```python
from build123d import *

# Parameters (mm, degrees)
SKETCH1_W                  = 120
SKETCH1_H                  = 50
BOSS_EXTRUDE1_DEPTH        = 160
SHELL1_T                   = -5
CUT_EXTRUDE2_REACH         = 174.699
SKETCH4_W                  = 72
SKETCH4_H                  = 39
SKETCH5_W                  = 80
SKETCH5_H                  = 43.5
CUT_EXTRUDE3_DEPTH         = 1
CUT_EXTRUDE4_REACH         = 174.699
SKETCH7_R                  = 10.054878977
CUT_EXTRUDE5_DEPTH         = 1
CUT_EXTRUDE6_REACH         = 203.556
SKETCH9_R                  = 1.35
CHAMFER1_SIZE              = 1.5
SKETCH10_W                 = 12
SKETCH10_H                 = 28
CUT_EXTRUDE7_DEPTH         = 2
LPATTERN1_COUNT            = 2
LPATTERN1_PITCH            = 50
CHAMFER1_OF_LPATTERN1_SIZE = 1.5
SKETCH11_W                 = 19.287715199
SKETCH11_H                 = 31.517777442
CUT_EXTRUDE8_DEPTH         = 202.556443707
SKETCH12_W                 = 24.096142941
SKETCH12_H                 = 37.033540034
CUT_EXTRUDE9_DEPTH         = 3
CUT_EXTRUDE10_REACH        = 174.699
SKETCH13_W                 = 24.602100194
SKETCH13_H                 = 34.536068778
SKETCH2_W                  = 80
SKETCH2_H                  = 57.520884572
CUT_EXTRUDE1_DEPTH         = 177.705970471


with BuildPart() as part:
    # Sketch1 → Boss-Extrude1 (new body)
    with BuildSketch(Plane.XY):
        Rectangle(SKETCH1_W, SKETCH1_H)
    extrude(amount=-BOSS_EXTRUDE1_DEPTH)

    # Shell1
    shell1_openings = [part.faces().sort_by_distance(p)[0] for p in [
        (-60, 0, -80),
        (0, 25, -80),
    ]]
    offset(amount=SHELL1_T, openings=shell1_openings, kind=Kind.INTERSECTION)

    # Sketch4 → Cut-Extrude2 (cut, up to next)
    with BuildSketch(Plane.XY, mode=Mode.PRIVATE) as cut_extrude2_sk1:
        with Locations((-7.752822836, -0.864806595)):
            Rectangle(SKETCH4_W, SKETCH4_H)
    cut_extrude2_tool1 = extrude(cut_extrude2_sk1.sketch, amount=-CUT_EXTRUDE2_REACH, mode=Mode.PRIVATE) & part.part
    add(cut_extrude2_tool1.solids().sort_by_distance((-7.752823, -0.864807, 0))[0], mode=Mode.SUBTRACT)

    # Sketch5 → Cut-Extrude3 (cut)
    with BuildSketch(Plane.XY):
        with Locations((-7.752822836, -0.864806595)):
            Rectangle(SKETCH5_W, SKETCH5_H)
    extrude(amount=-CUT_EXTRUDE3_DEPTH, mode=Mode.SUBTRACT)

    # Sketch6 → Cut-Extrude4 (cut, up to next)
    with BuildSketch(Plane.XY, mode=Mode.PRIVATE) as cut_extrude4_sk1:
        with BuildLine():
            Line((51.25624878, 9.193705725), (51.25624878, 16.439437846))
            ThreePointArc((51.25624878, 16.439437846), (44.123588582, 20.816571785), (36.990928383, 16.439437846))
            Line((36.990928383, 16.439437846), (36.990928383, 9.193705725))
            ThreePointArc((36.990928383, 9.193705725), (44.123588582, 4.816571785), (51.25624878, 9.193705725))
        make_face()
    cut_extrude4_tool1 = extrude(cut_extrude4_sk1.sketch, amount=-CUT_EXTRUDE4_REACH, mode=Mode.PRIVATE) & part.part
    cut_extrude4 = cut_extrude4_tool1.solids().sort_by_distance((44.123589, 12.816572, 0))[0]
    add(cut_extrude4, mode=Mode.SUBTRACT)

    # Sketch7 → Cut-Extrude5 (cut)
    with BuildSketch(Plane.XY):
        with Locations((44.123588582, 12.816571785)):
            Circle(SKETCH7_R)
    cut_extrude5 = extrude(amount=-CUT_EXTRUDE5_DEPTH, mode=Mode.SUBTRACT)

    # Mirror1: Cut-Extrude4, Cut-Extrude5 mirrored; each copy of Cut-Extrude4 runs up to whatever stops it at its own place
    mirror1_before = part.part  # the part as the pattern finds it: every copy runs up to it
    mirror1_cut_extrude4_long = extrude(cut_extrude4_sk1.sketch, amount=-CUT_EXTRUDE4_REACH, mode=Mode.PRIVATE)
    mirror1_cut_extrude4_tool = mirror1_cut_extrude4_long.mirror(Plane.ZX) & mirror1_before
    add(mirror1_cut_extrude4_tool.solids().sort_by_distance((44.123589, -12.816572, 0))[0], mode=Mode.SUBTRACT)
    add(cut_extrude5.mirror(Plane.ZX), mode=Mode.SUBTRACT)

    # Sketch9 → Cut-Extrude6 (cut, up to next)
    with BuildSketch(Plane(origin=(60, 0, 0), x_dir=(0, 0, -1), z_dir=(1, 0, 0)), mode=Mode.PRIVATE) as cut_extrude6_sk1:
        with Locations((34.250404533, 14.202757041)):
            Circle(SKETCH9_R)
    cut_extrude6_tool1 = extrude(cut_extrude6_sk1.sketch, amount=-CUT_EXTRUDE6_REACH, mode=Mode.PRIVATE) & part.part
    # Sketch9 → Cut-Extrude6 (cut, up to next)
    with BuildSketch(Plane(origin=(60, 0, 0), x_dir=(0, 0, -1), z_dir=(1, 0, 0)), mode=Mode.PRIVATE) as cut_extrude6_sk2:
        with Locations((34.250404533, -8.297242959)):
            Circle(SKETCH9_R)
    cut_extrude6_tool2 = extrude(cut_extrude6_sk2.sketch, amount=-CUT_EXTRUDE6_REACH, mode=Mode.PRIVATE) & part.part
    # Sketch9 → Cut-Extrude6 (cut, up to next)
    with BuildSketch(Plane(origin=(60, 0, 0), x_dir=(0, 0, -1), z_dir=(1, 0, 0)), mode=Mode.PRIVATE) as cut_extrude6_sk3:
        with BuildLine():
            Line((29.950404533, -5.047242959), (38.550404533, -5.047242959))
            Line((38.550404533, -5.047242959), (38.550404533, 7.952757041))
            ThreePointArc((38.550404533, 7.952757041), (37.671724876, 10.074077384), (35.550404533, 10.952757041))
            Line((35.550404533, 10.952757041), (32.950404533, 10.952757041))
            ThreePointArc((32.950404533, 10.952757041), (30.829084189, 10.074077384), (29.950404533, 7.952757041))
            Line((29.950404533, 7.952757041), (29.950404533, -5.047242959))
        make_face()
    cut_extrude6_tool3 = extrude(cut_extrude6_sk3.sketch, amount=-CUT_EXTRUDE6_REACH, mode=Mode.PRIVATE) & part.part
    cut_extrude6_1 = cut_extrude6_tool1.solids().sort_by_distance((60, 14.202757, -34.250405))[0]
    add(cut_extrude6_1, mode=Mode.SUBTRACT)
    cut_extrude6_2 = cut_extrude6_tool2.solids().sort_by_distance((60, -8.297243, -34.250405))[0]
    add(cut_extrude6_2, mode=Mode.SUBTRACT)
    cut_extrude6_3 = cut_extrude6_tool3.solids().sort_by_distance((60, 2.741042, -34.250405))[0]
    add(cut_extrude6_3, mode=Mode.SUBTRACT)
    cut_extrude6 = cut_extrude6_1 + cut_extrude6_2 + cut_extrude6_3  # Cut-Extrude6 as one shape, for the pattern or mirror that repeats it

    # Chamfer1
    chamfer1_edges = [part.edges().sort_by_distance(p)[0] for p in [
        (60, -8.297242959, -32.900404533),
        (60, 14.202757041, -32.900404533),
    ]]
    chamfer(chamfer1_edges, length=CHAMFER1_SIZE)

    # Sketch10 → Cut-Extrude7 (cut)
    with BuildSketch(Plane.ZY.offset(-55)):
        with Locations((-34.250404533, 2.952757041)):
            Rectangle(SKETCH10_W, SKETCH10_H)
    cut_extrude7 = extrude(amount=-CUT_EXTRUDE7_DEPTH, mode=Mode.SUBTRACT)

    # LPattern1: Cut-Extrude6, Cut-Extrude7 ×2
    with Locations(*[(0, 0, -i * LPATTERN1_PITCH) for i in range(1, LPATTERN1_COUNT)]):
        add(cut_extrude6, mode=Mode.SUBTRACT)
        add(cut_extrude7, mode=Mode.SUBTRACT)

    # Chamfer1 of LPattern1
    chamfer1_of_lpattern1_edges = [part.edges().sort_by_distance(p)[0] for p in [
        (60, -8.297242959, -82.900404533),
        (60, 14.202757041, -82.900404533),
    ]]
    chamfer(chamfer1_of_lpattern1_edges, length=CHAMFER1_OF_LPATTERN1_SIZE)

    # Sketch11 → Cut-Extrude8 (cut, through all)
    with BuildSketch(Plane(origin=(60, 0, 0), x_dir=(0, 0, -1), z_dir=(1, 0, 0))):
        with Locations((111.274658912, 0)):
            Rectangle(SKETCH11_W, SKETCH11_H)
    extrude(amount=-CUT_EXTRUDE8_DEPTH, mode=Mode.SUBTRACT)

    # Sketch12 → Cut-Extrude9 (cut)
    with BuildSketch(Plane(origin=(60, 0, 0), x_dir=(0, 0, -1), z_dir=(1, 0, 0))):
        with Locations((111.274658912, 0)):
            Rectangle(SKETCH12_W, SKETCH12_H)
    extrude(amount=-CUT_EXTRUDE9_DEPTH, mode=Mode.SUBTRACT)

    # Sketch13 → Cut-Extrude10 (cut, up to next)
    with BuildSketch(Plane(origin=(0, 0, -160), x_dir=(-1, 0, 0), z_dir=(0, 0, -1)), mode=Mode.PRIVATE) as cut_extrude10_sk1:
        with Locations((-30.86599902, 0)):
            Rectangle(SKETCH13_W, SKETCH13_H)
    cut_extrude10_tool1 = extrude(cut_extrude10_sk1.sketch, amount=-CUT_EXTRUDE10_REACH, mode=Mode.PRIVATE) & part.part
    add(cut_extrude10_tool1.solids().sort_by_distance((30.865999, 0, -160))[0], mode=Mode.SUBTRACT)

    # Sketch2 → Cut-Extrude1 (cut, through all)
    with BuildSketch(Plane(origin=(0, -20, 0), x_dir=(1, 0, 0), z_dir=(0, 1, 0))):
        with Locations((-20, 183.760442286)):
            Rectangle(SKETCH2_W, SKETCH2_H)
    extrude(amount=CUT_EXTRUDE1_DEPTH, mode=Mode.SUBTRACT)


solid = part.part
```
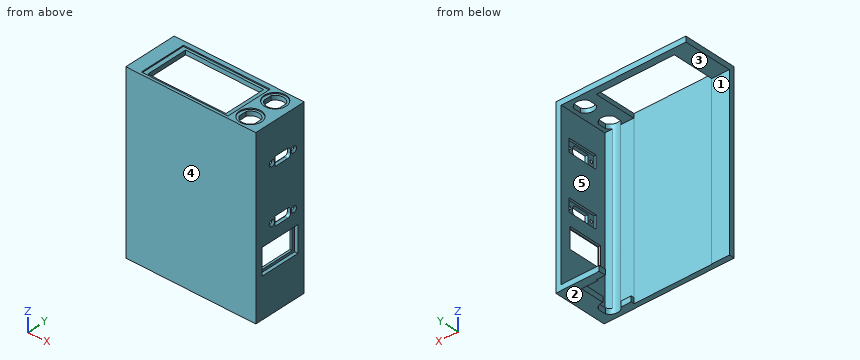
Geometry: final body of the model. Coordinates: model frame, mm. Face numbers are marked on the shaded views. A direction names the side the tool comes from. Give positions to 0.01 mm unless a question says otherwise; leave off trailing zeros. Order: outer loops, then holes, each group sorted by start corner. A loop starts at its lowest first (then second) coordinate and runs counter-clockwise, first axis right, second up. Notation, with made-up numbers: (-35, 58) -> (-27, 58) arc R22 cw to (-27, 88) -> close; hole circle Ø1 at (59, 13.5). An arc over 180 degrees is marked (long way). Write each question's results on one line, items separated by ' | '. Start each with the question number.
1) Section D-D (z = -16). Return loops of the section in (x, y).
2) Section A-A (z = -118). Return loops of the section in (x, y).
3) First-contact query: pin 1 (5.5 mm diameter, centred on y = 4, z = -157.5, fed in from -X); pin 2 (8 mm diameter, centred on x = 16, y = 17.5, fed in from -Z); pin 3 (1 mm diameter, centred on y = -1, z = -100, fed in from -X). Flat tips, straight axial feed; report the tip coordinate or a pass-through.
4) Line query: line 1 (Z direction, x = 51, y = 8.5); line 2 (Z direction, x = 52, y = 2); line 3 (X direction, y = 8.5, z = -54). Output: solid intervals per line, ascending. Write a range as from..to.
5) Set-up query: the marked faces 4 and 5. Return all of +Z, -Z, +X, -X, +Y, -Y with unobstructed straight access to the full face (end or side cutting, diameter ignored); none if empty.
6) Draft query along Z for the marked faces 1, 2 and 3. Return one class per face: pulls with the +Z half, pulls with the -Z half, needs draft (parallel to the pull), parting line crosses it, or undercut.
7) Section C-C (x = 49.5). Return loops of the section in (y, z), then the cut area to 3 significant figures.
8) Section B-B (x = 15.5). Return loops of the section in (y, z).
Calculated:
1) outline: (-60, -25) -> (60, -25) -> (60, 25) -> (55, 25) -> (55, -20) -> (47.64, -20) arc R8 cw to (40.6, -20) -> (28.25, -20) -> (28.25, -20.36) -> (-43.75, -20.36) -> (-43.75, -20) -> (-60, -20) -> close
2) outline: (-60, -25) -> (60, -25) -> (60, -18.52) -> (57, -18.52) -> (57, -15.76) -> (55, -15.76) -> (55, -20) -> (47.64, -20) arc R8 cw to (40.6, -20) -> (28.25, -20) -> (28.25, -20.36) -> (-43.75, -20.36) -> (-43.75, -20) -> (-60, -20) -> close; (55, 15.76) -> (57, 15.76) -> (57, 18.52) -> (60, 18.52) -> (60, 25) -> (55, 25) -> close
3) pin 1: x = 43.17 | pin 2: z = -5 | pin 3: x = 55
4) line 1: -160..-155, -5..-1 | line 2: -160..-155, -5..0 | line 3: 55..60
5) face 4: +Z, -Z, +X, -X, -Y | face 5: -X, +Y
6) face 1: needs draft | face 2: pulls with the -Z half | face 3: undercut
7) outline: (-25, -160) -> (-18.74, -160) -> (-18.74, -155) -> (-20, -155) -> (-20, -5) -> (-18.74, -5) -> (-18.74, -1) -> (-21.31, -1) -> (-21.31, 0) -> (-25, 0) -> close; (-6.89, -160) -> (25, -160) -> (25, -155) -> (-6.89, -155) -> close; (-6.89, -5) -> (6.89, -5) -> (6.89, -1) -> (4.32, -1) -> (4.32, 0) -> (-4.32, 0) -> (-4.32, -1) -> (-6.89, -1) -> close; (18.74, -5) -> (25, -5) -> (25, 0) -> (21.31, 0) -> (21.31, -1) -> (18.74, -1) -> close | area: 1,060 mm2
8) outline: (-25, -160) -> (-20.36, -160) -> (-20.36, -1) -> (-22.61, -1) -> (-22.61, 0) -> (-25, 0) -> close; (18.64, -5) -> (25, -5) -> (25, 0) -> (20.89, 0) -> (20.89, -1) -> (18.64, -1) -> close
